The listing builds one solid part. Answer for the finished solid, in the listing's coordinates (mm). Face numbers are marked on the shaded views. A direction names the side the tool comes from. Coordinates: 2 decimals unless noted, no trailing zeros. Order: outer loops, then holes, each group sorted by start corner. A loop starts at its lowest first (then second) coordinate and runs counter-clockwise, first axis right, second up. Notation, with made-up numbers: (10.5, -38.5) -> (61.5, -38.5) arc R32 cw to (61.5, -11.5) -> close; hole circle Ø1 at (12.25, 5.25). An arc over 180 degrees is marked (long way). Put each result on its own line as item: value. Start each with the question number.
```python
from build123d import *

# Parameters (mm, degrees)
CHAMFER_1_SIZE      = 5
CUT_EXTRUDE_START   = 33.5
CUT_EXTRUDE_1_DEPTH = 129.093626112


with BuildPart() as part:
    # Эскиз1 → Повернуть1 (revolve)
    with BuildSketch(Plane.XY, mode=Mode.PRIVATE) as revolve_1_sk:
        Polygon((-70, 0), (-70, 25), (0, 25), (0, 42.5), (100, 42.5), (100, 25), (150, 25), (150, 0), align=None)
    revolve(revolve_1_sk.sketch.rotate(Axis((0, 0, 0), (1, 0, 0)), 90), axis=Axis((0, 0, 0), (1, 0, 0)))

    # Фаска1
    chamfer_1_edges = [part.edges().sort_by_distance(p)[0] for p in [
        (150, 0, -25),
        (0, 0, -42.5),
        (-70, 0, -25),
    ]]
    chamfer(chamfer_1_edges, length=CHAMFER_1_SIZE)

    # Эскиз2 → Вырез-Повернуть1 (revolve, cut)
    with BuildSketch(Plane.XY, mode=Mode.PRIVATE) as cut_revolve_1_sk:
        with BuildLine():
            Line((0, 25), (0, 24.5))
            ThreePointArc((0, 24.5), (-0.585786438, 23.085786438), (-2, 22.5))
            Line((-2, 22.5), (-5.085786438, 22.5))
            ThreePointArc((-5.085786438, 22.5), (-5.46846987, 22.576120467), (-5.792893219, 22.792893219))
            Line((-5.792893219, 22.792893219), (-8, 25))
            Line((-8, 25), (0, 25))
        make_face()
    revolve(cut_revolve_1_sk.sketch.rotate(Axis((0, 0, 0), (1, 0, 0)), 90), axis=Axis((0, 0, 0), (1, 0, 0)), mode=Mode.SUBTRACT)

    # Эскиз3 → Вырез-Вытянуть1 (cut, through all)
    with BuildSketch(Plane(origin=(0, 0, 0), x_dir=(1, 0, 0), z_dir=(0, 1, 0)).offset(CUT_EXTRUDE_START)):
        with BuildLine():
            Line((28.5, 11), (76.5, 11))
            ThreePointArc((76.5, 11), (87.5, 0), (76.5, -11))
            Line((76.5, -11), (28.5, -11))
            ThreePointArc((28.5, -11), (17.5, 0), (28.5, 11))
        make_face()
    extrude(amount=CUT_EXTRUDE_1_DEPTH, mode=Mode.SUBTRACT)

    # Эскиз4 → Вырез-Повернуть3 (revolve, cut)
    with BuildSketch(Plane(origin=(125, 0, 0), x_dir=(0, 0, -1), z_dir=(1, 0, 0))):
        Polygon((-10, 0), (-14.041451884, 7), (-25, 7), (-25, 0), align=None)
    revolve(axis=Axis((125, 0, 10), (0, 0, 1)), mode=Mode.SUBTRACT)


solid = part.part
```
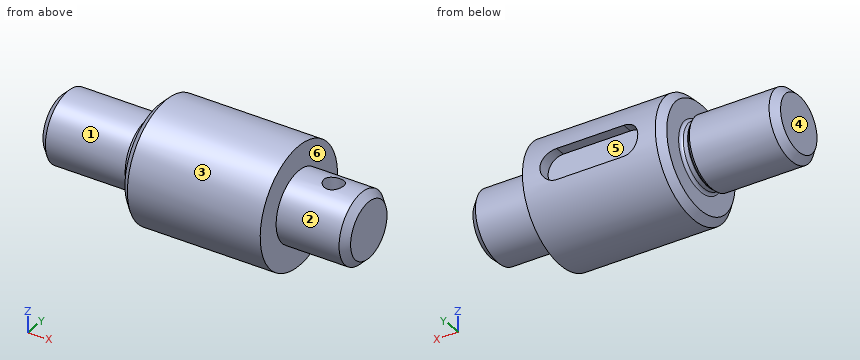
(1) The part is cut by section C-C on x = 72.5. Determine the outline of the cut face in (y, z), plus the area to 3 significant figures.
(2) The part is cut by section B-B on x = -38.5. Determine the outline of the cut face in (y, z), plus the area to 3 significant figures.
(3) Each of these flat-tipped pins is pushed along its axis until it touches: P1, Ø2, axis at y = 19.5, z = -22.5, coming from the +X side; P2, Ø8.5, axis at x = 44.5, y = 37.5, coming from the -Z side; P3, Ø4, axis at x = 75.5, y = 12, coming from the -Z side. Where does it stop, or does it pass through?
(4) Find the intervals of material crossed by L1, parallel to X at y = 0, z = 18; L2, parallel to X at y = 13, z = -27; L3, parallel to Z at x = 9.5, y = -1, in increasing order.
(5) For a pull along X with two mould halves and no side action, classify the marked faces 4, 5 and 6 as released by +X, released by -X, zero draft, split by the parting line, or undercut.
(6) A tool of negligible diameter and unlimited length cuts with its end or side. For the marked faces 1, 2 and 3, from which of +Z, -Z, +X, -X, +Y, -Y can it reach the whole face along a straight path? Write none if from no direction.
Worked out:
1. outline: (33.5, -11) -> (33.5, 11) -> (41.05, 11) arc R42.5 ccw (long way) to (41.05, -11) -> close
1. area: 5,490 mm2
2. outline: circle Ø50 at (0, 0)
2. area: 1,960 mm2
3. P1: x = 100
3. P2: z = -26.47
3. P3: z = -41.31
4. L1: -70 to 118, 132 to 150
4. L2: 0 to 100
4. L3: -42.49 to 42.49
5. face 4: released by -X
5. face 5: undercut
5. face 6: released by +X
6. face 1: -X
6. face 2: +X
6. face 3: +X, -X
